Could you check a few things on this model? Use its own coordinates, in mm. Face numbers are marked on the shaded views. Give positions to 0.01 mm unless a question says otherwise; leave off trailing zeros. Loops run counter-clockwise (first coordinate to the right, second up) from the corner with the lowest first, then second, coordinate; pieces in that order, holes last. Notation, with made-up numbers: M -6.75,20.5 L 36.25,20.5 A23 cw 36.25,39.5 Z; hole C 33.25,-20.5 d2. An arc over 180 degrees is marked long. Use a Markdown table: item, result. Add a question column.
1) Suppose I cut it at A-A on x = 0. List the corners of the cut face in (y, z) for me, and give its area (3 significant figures).
2) Will these pins go through, and if not, where does the flat tip stop? pin 1 Ø3 at (x, y) = (0, -2) entering from +Z; pin 2 Ø4 at (x, z) = (-1, 142.5) entering from +Y; pin 3 Ø4 at (y, z) = (3.5, 143.5) entering from +X; pin 4 Ø4 at (y, z) = (0, 143) entering from -X.
3) We'd pull the mould along Z, two halves only. Please class the marked faces 1, 2 and 3: +Z half, -Z half, draft (parallel to the pull), parting line (faces both ways), or undercut.
4) Suppose I cut it at C-C on z = 15.5. List the corners of the cut face in (x, y) for me, and give its area (3 significant figures).
5) Suppose I cut it at B-B on y = 0. List the corners of the cut face in (x, z) for me, and give its area (3 significant figures).
6) If I drill on line 1 along Y through (x, z) = (0, 90); line 2 along Z through (x, y) = (-2, 14); line 3 along X through (y, z) = (-0.5, 77), over which ranges is the centre line in solid material (lowest first)? Write a range as [from, to].
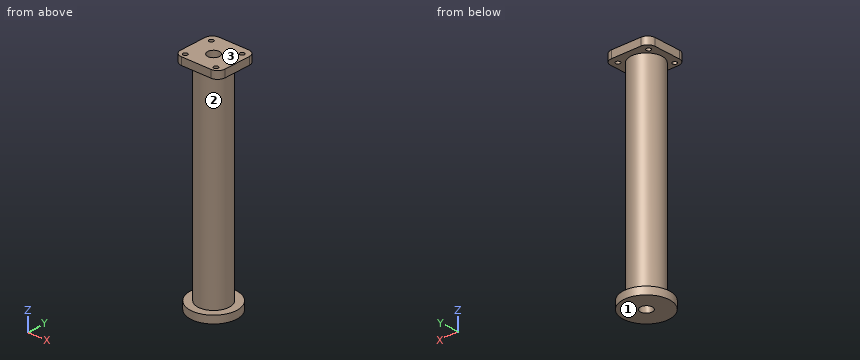
```python
from build123d import *

# Parameters (mm, degrees)
SKETCH1_R           = 10.5
SKETCH1_R_2         = 4
BOSS_EXTRUDE1_DEPTH = 140
SKETCH2_W           = 30
SKETCH2_H           = 28
SKETCH2_R           = 1.5
SKETCH2_R_2         = 4
BOSS_EXTRUDE2_DEPTH = 5
FILLET1_R           = 5
SKETCH3_R           = 15.5
SKETCH3_R_2         = 10.5
EXTRUDE_THIN1_DEPTH = 5


with BuildPart() as part:
    # Sketch1 → Boss-Extrude1 (new body)
    with BuildSketch(Plane.XY):
        Circle(SKETCH1_R)
        Circle(SKETCH1_R_2, mode=Mode.SUBTRACT)
    extrude(amount=BOSS_EXTRUDE1_DEPTH)

    # Sketch2 → Boss-Extrude2 (add)
    with BuildSketch(Plane.XY.offset(140)):
        with Locations((0, 1)):
            Rectangle(SKETCH2_W, SKETCH2_H)
        with Locations((-10.388295362, 9.695742338)):
            Circle(SKETCH2_R, mode=Mode.SUBTRACT)
        with Locations((10.388295362, -9.695742338)):
            Circle(SKETCH2_R, mode=Mode.SUBTRACT)
        with Locations((10.388295362, 9.695742338)):
            Circle(SKETCH2_R, mode=Mode.SUBTRACT)
        with Locations((-10.388295362, -9.695742338)):
            Circle(SKETCH2_R, mode=Mode.SUBTRACT)
        Circle(SKETCH2_R_2, mode=Mode.SUBTRACT)
    extrude(amount=BOSS_EXTRUDE2_DEPTH)

    # Fillet1
    fillet1_edges = [part.edges().sort_by_distance(p)[0] for p in [
        (15, -13, 142.5),
        (15, 15, 142.5),
        (-15, 15, 142.5),
        (-15, -13, 142.5),
    ]]
    fillet(fillet1_edges, radius=FILLET1_R)

    # Sketch3 → Extrude-Thin1 (add)
    with BuildSketch(Plane(origin=(0, 0, 0), x_dir=(-1, 0, 0), z_dir=(0, 0, -1))):
        Circle(SKETCH3_R)
        Circle(SKETCH3_R_2, mode=Mode.SUBTRACT)
    extrude(amount=-EXTRUDE_THIN1_DEPTH)


solid = part.part
```
Answer block:
| question | item | result |
|---|---|---|
| 1 | outline | M -15.5,0 L -4,0 L -4,145 L -13,145 L -13,140 L -10.5,140 L -10.5,5 L -15.5,5 Z; M 4,0 L 15.5,0 L 15.5,5 L 10.5,5 L 10.5,140 L 15,140 L 15,145 L 4,145 Z |
| 1 | area | 1,970 mm^2 |
| 2 | pin 1 | passes through |
| 2 | pin 2 | stops at y = 15 |
| 2 | pin 3 | stops at x = 15 |
| 2 | pin 4 | stops at x = -15 |
| 3 | face 1 | -Z half |
| 3 | face 2 | undercut |
| 3 | face 3 | +Z half |
| 4 | outline | C 0,0 d21; hole C 0,0 d8 |
| 4 | area | 296 mm^2 |
| 5 | outline | M -15.5,0 L -4,0 L -4,145 L -15,145 L -15,140 L -10.5,140 L -10.5,5 L -15.5,5 Z; M 4,0 L 15.5,0 L 15.5,5 L 10.5,5 L 10.5,140 L 15,140 L 15,145 L 4,145 Z |
| 5 | area | 1,980 mm^2 |
| 6 | line 1 | y = [-10.5, -4], [4, 10.5] |
| 6 | line 2 | z = [0, 5], [140, 145] |
| 6 | line 3 | x = [-10.49, -3.97], [3.97, 10.49] |
